from build123d import *

# Parameters (mm, degrees)
SKETCH1_R           = 7.5
BOSS_EXTRUDE1_DEPTH = 115
CHAMFER1_SIZE       = 1


with BuildPart() as part:
    # Sketch1 → Boss-Extrude1 (new body)
    with BuildSketch(Plane(origin=(0, 0, 0), x_dir=(1, 0, 0), z_dir=(0, 1, 0))):
        with Locations(Location((0, 0, 0), (0, 0, 270))):
            Circle(SKETCH1_R)
    extrude(amount=BOSS_EXTRUDE1_DEPTH)

    # Sketch2 → Cut-Revolve1 (revolve, cut)
    with BuildSketch(Plane.XY, mode=Mode.PRIVATE) as cut_revolve1_sk:
        with BuildLine():
            Line((-3.618601574, 112.704618035), (-3.618601574, 116.762708117))
            Line((-3.618601574, 116.762708117), (0, 116.762708117))
            Line((0, 116.762708117), (0, 115))
            ThreePointArc((0, 115), (-2.142606807, 114.37775607), (-3.618601574, 112.704618035))
        make_face()
    revolve(cut_revolve1_sk.sketch.rotate(Axis((0, 125.515236919, 0), (0, -1, 0)), 270), axis=Axis((0, 125.515236919, 0), (0, -1, 0)), mode=Mode.SUBTRACT)

    # Chamfer1
    chamfer1_edges = [part.edges().sort_by_distance(p)[0] for p in [
        (0, 115, -7.5),
        (0, 115, -3.618601574),
    ]]
    chamfer(chamfer1_edges, length=CHAMFER1_SIZE)


solid = part.part
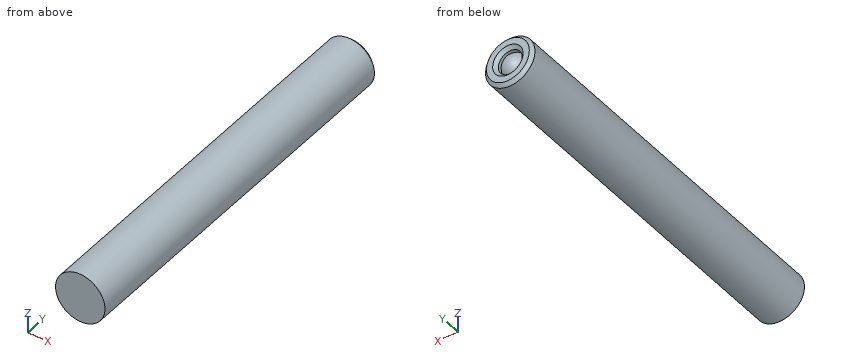
Could you check a few things on this model? Use its own coordinates, in mm. Round coordinates to 2 decimals unless told otherwise and drop trailing zeros. Order: outer loops, then holes, each group sorted by start corner. A loop starts at its lowest first (then second) coordinate and runs counter-clockwise, first axis right, second up.
Q1. I'm going to push flat-ended pins straight in: P1, Ø1.5, axis at x = 3.5, y = 93.5, coming from the +Z side; P2, Ø5, axis at y = 27.5, z = 5.5, coming from the +X side; P3, Ø4, axis at y = 23.5, z = 2.5, coming from the -X side. Where does each tip first touch, or does it pass through?
Geometry says:
P1: stops at z = 6.98
P2: stops at x = 6.87
P3: stops at x = -7.48
Q2. Imagine slicing it at A-A, the plane y = 9. List the corners of the cut face in (x, z) for me, then the cut area to 3 significant figures.
Geometry says:
outline: circle Ø15 at (0, 0)
area: 177 mm2
Q3. Please list where these lines run through material, in increasing order: probe 1 along X at (y, z) = (113.6, 0); probe 2 along X at (y, z) = (113.5, 0); probe 3 along Z at (x, y) = (3.75, 44.5).
Geometry says:
probe 1: x = -7.5 to -3.62, -3.04 to 3.04, 3.62 to 7.5
probe 2: x = -7.5 to -3.62, -3.12 to 3.12, 3.62 to 7.5
probe 3: z = -6.5 to 6.5
